```python
from build123d import *

# Parameters (mm, degrees)
EXTRUDE_1_DEPTH = 299.99673285
CHAMFER_1_SIZE  = 1
CHAMFER_2_SIZE  = 1
FILLET_1_R      = 0.5
FILLET_2_R      = 0.5
FILLET_3_R      = 0.5
FILLET_4_R      = 0.5
FILLET_5_R      = 0.5
FILLET_6_R      = 0.5
FILLET_7_R      = 0.5
CHAMFER_4_SIZE  = 1
CHAMFER_5_SIZE  = 1


with BuildPart() as part:
    # Эскиз1 → Бобышка-Вытянуть1 (new body)
    with BuildSketch(Plane.XY):
        with BuildLine():
            Line((-1.25, 0), (-1.25, 6.869523989))
            ThreePointArc((-1.25, 6.869523989), (0, 8.9), (1.25, 6.869523989))
            Line((1.25, 6.869523989), (1.25, 0))
            Line((1.25, 0), (4, 0))
            Line((4, 0), (4, 2))
            Line((4, 2), (6, 4))
            Line((6, 4), (6, 25.25))
            Line((6, 25.25), (21, 25.25))
            Line((21, 25.25), (21, 27.75))
            Line((21, 27.75), (6, 27.75))
            Line((6, 27.75), (6, 29.65))
            Line((6, 29.65), (21, 29.65))
            Line((21, 29.65), (21, 32.15))
            Line((21, 32.15), (6, 32.15))
            Line((6, 32.15), (6, 34.05))
            Line((6, 34.05), (21, 34.05))
            Line((21, 34.05), (21, 36.55))
            Line((21, 36.55), (6, 36.55))
            Line((6, 36.55), (6, 38.45))
            Line((6, 38.45), (21, 38.45))
            Line((21, 38.45), (21, 40.95))
            Line((21, 40.95), (6, 40.95))
            Line((6, 40.95), (6, 42.85))
            Line((6, 42.85), (21, 42.85))
            Line((21, 42.85), (21, 45.35))
            Line((21, 45.35), (6, 45.35))
            Line((6, 45.35), (6, 47.25))
            Line((6, 47.25), (21, 48))
            Line((21, 48), (21, 49))
            Line((21, 49), (1.25, 49))
            Line((1.25, 49), (1.25, 42.116940633))
            ThreePointArc((1.25, 42.116940633), (0, 40.106043134), (-1.25, 42.116940633))
            Line((-1.25, 42.116940633), (-1.25, 49))
            Line((-1.25, 49), (-14, 49))
            Line((-14, 49), (-14, 46.65))
            Line((-14, 46.65), (-4, 46.65))
            Line((-4, 46.65), (-4, 43.95))
            Line((-4, 43.95), (-14, 43.95))
            Line((-14, 43.95), (-14, 42.25))
            Line((-14, 42.25), (-4, 42.25))
            Line((-4, 42.25), (-4, 39.55))
            Line((-4, 39.55), (-14, 39.55))
            Line((-14, 39.55), (-14, 37.85))
            Line((-14, 37.85), (-4, 37.85))
            Line((-4, 37.85), (-4, 35.15))
            Line((-4, 35.15), (-9, 35.15))
            Line((-9, 35.15), (-9, 33.45))
            Line((-9, 33.45), (-4, 33.45))
            Line((-4, 33.45), (-4, 0))
            Line((-4, 0), (-1.25, 0))
        make_face()
    extrude(amount=EXTRUDE_1_DEPTH)

    # Фаска1
    chamfer_1_edges = [part.edges().sort_by_distance(p)[0] for p in [
        (-1.25, 0, 149.998366425),
    ]]
    chamfer(chamfer_1_edges, length=CHAMFER_1_SIZE)

    # Фаска2
    chamfer_2_edges = [part.edges().sort_by_distance(p)[0] for p in [
        (1.25, 0, 149.998366425),
    ]]
    chamfer(chamfer_2_edges, length=CHAMFER_2_SIZE)

    # Скругление1
    fillet_1_edges = [part.edges().sort_by_distance(p)[0] for p in [
        (-9, 33.45, 149.998366425),
        (-9, 35.15, 149.998366425),
        (-14, 37.85, 149.998366425),
        (-14, 39.55, 149.998366425),
        (-14, 42.25, 149.998366425),
        (-14, 43.95, 149.998366425),
        (-14, 46.65, 149.998366425),
    ]]
    fillet(fillet_1_edges, radius=FILLET_1_R)

    # Скругление2
    fillet_2_edges = [part.edges().sort_by_distance(p)[0] for p in [
        (-4, 35.15, 149.998366425),
        (-4, 39.55, 149.998366425),
        (-4, 43.95, 149.998366425),
    ]]
    fillet(fillet_2_edges, radius=FILLET_2_R)

    # Скругление3
    fillet_3_edges = [part.edges().sort_by_distance(p)[0] for p in [
        (-4, 37.85, 149.998366425),
        (-4, 42.25, 149.998366425),
        (-4, 46.65, 149.998366425),
    ]]
    fillet(fillet_3_edges, radius=FILLET_3_R)

    # Скругление4
    fillet_4_edges = [part.edges().sort_by_distance(p)[0] for p in [
        (-14, 49, 149.998366425),
    ]]
    fillet(fillet_4_edges, radius=FILLET_4_R)

    # Скругление5
    fillet_5_edges = [part.edges().sort_by_distance(p)[0] for p in [
        (21, 49, 149.998366425),
        (21, 48, 149.998366425),
        (21, 45.35, 149.998366425),
        (21, 42.85, 149.998366425),
        (21, 40.95, 149.998366425),
        (21, 38.45, 149.998366425),
        (21, 36.55, 149.998366425),
        (21, 34.05, 149.998366425),
        (21, 32.15, 149.998366425),
        (21, 29.65, 149.998366425),
        (21, 27.75, 149.998366425),
        (21, 25.25, 149.998366425),
    ]]
    fillet(fillet_5_edges, radius=FILLET_5_R)

    # Скругление6
    fillet_6_edges = [part.edges().sort_by_distance(p)[0] for p in [
        (6, 47.25, 149.998366425),
        (6, 42.85, 149.998366425),
        (6, 38.45, 149.998366425),
        (6, 34.05, 149.998366425),
        (6, 29.65, 149.998366425),
    ]]
    fillet(fillet_6_edges, radius=FILLET_6_R)

    # Скругление7
    fillet_7_edges = [part.edges().sort_by_distance(p)[0] for p in [
        (6, 45.35, 149.998366425),
        (6, 40.95, 149.998366425),
        (6, 36.55, 149.998366425),
        (6, 32.15, 149.998366425),
        (6, 27.75, 149.998366425),
    ]]
    fillet(fillet_7_edges, radius=FILLET_7_R)

    # Фаска4
    chamfer_4_edges = [part.edges().sort_by_distance(p)[0] for p in [
        (-1.25, 49, 149.998366425),
    ]]
    chamfer(chamfer_4_edges, length=CHAMFER_4_SIZE)

    # Фаска5
    chamfer_5_edges = [part.edges().sort_by_distance(p)[0] for p in [
        (1.25, 49, 149.998366425),
    ]]
    chamfer(chamfer_5_edges, length=CHAMFER_5_SIZE)


solid = part.part
```
For this review, take the finished solid that the model builds, in its own axes (mm). A direction names the side the tool comes from. Round coordinates to 2 decimals unless told otherwise and drop trailing zeros. Loops run counter-clockwise (first coordinate to the right, second up) from the corner with the lowest first, then second, coordinate; pieces in that order, holes last.
Q1. To check wall thickness, follow line 1 along Y through (x, z) = (-9.5, 263); line 2 along Y through (x, z) = (17, 187); line 3 along Y through (x, z) = (15.5, 285.5) (3 decimals). State the ranges of each line that lie inside material, in increasing order.
Result sheet:
line 1: y = 37.85 to 39.55, 42.25 to 43.95, 46.65 to 49
line 2: y = 25.25 to 27.75, 29.65 to 32.15, 34.05 to 36.55, 38.45 to 40.95, 42.85 to 45.35, 47.8 to 49
line 3: y = 25.25 to 27.75, 29.65 to 32.15, 34.05 to 36.55, 38.45 to 40.95, 42.85 to 45.35, 47.725 to 49
Q2. Insertion check: pin 1 Ø10 at (y, z) = (10, 259) entering from +X; pin 2 Ø0.8 at (y, z) = (45, 79) entering from -X; pin 3 Ø4 at (x, z) = (13.5, 193.5) entering from -Y. Each pin has a flat end and moves straight along its axis. Give the tip position at first contact, or say it passes through.
Result sheet:
pin 1: stops at x = 6
pin 2: stops at x = -4
pin 3: stops at y = 25.25
Q3. Add section A-A on x = 17. Write out the cut boundary in (y, z), plus the area to 3 significant figures.
Result sheet:
outline: (25.25, 0) - (27.75, 0) - (27.75, 300) - (25.25, 300) - close; (29.65, 0) - (32.15, 0) - (32.15, 300) - (29.65, 300) - close; (34.05, 0) - (36.55, 0) - (36.55, 300) - (34.05, 300) - close; (38.45, 0) - (40.95, 0) - (40.95, 300) - (38.45, 300) - close; (42.85, 0) - (45.35, 0) - (45.35, 300) - (42.85, 300) - close; (47.8, 0) - (49, 0) - (49, 300) - (47.8, 300) - close
area: 4,110 mm2
Q4. Add section B-B on y = 17. Write out the cut boundary in (x, z), plus the area to 3 significant figures.
Result sheet:
outline: (-4, 0) - (6, 0) - (6, 300) - (-4, 300) - close
area: 3,000 mm2
Q5. Mouldability with a two-part tool opening along X and no side actions: class faces 1 (the face through (-1.25, 4, 148)), 2 (the face through (-9, 37.85, 148)), 3 (the face through (1.25, 45, 148)) as +X half, -X half, draft (parallel to the pull), parting line (faces both ways), or undercut.
Result sheet:
face 1: undercut
face 2: draft
face 3: undercut
Q6. Machinability: for faces 4 (the face through (14, 27.75, 148)), 5 (the face through (-9, 42.25, 148)), 6 (the face through (13, 25.25, 148)), which of the approach directions +Z, -Z, +X, -X, +Y, -Y give a long, thin tool a straight path to every point of the face, cutting with its end or side? Answer none if there is none.
Result sheet:
face 4: +Z, -Z, +X
face 5: +Z, -Z, -X
face 6: +Z, -Z, +X, -Y
